Check sheet for the modelled part. Datum: model origin and axes. Units: mm. Face numbers are marked on the shaded views. A direction names the side the tool comes from. Round coordinates to 2 decimals unless told otherwise and drop trailing zeros. Order: outer loops, then holes, each group sorted by start corner. A loop starts at its lowest first (then second) coordinate and runs counter-clockwise, first axis right, second up.
```python
from build123d import *

# Parameters (mm, degrees)
SKETCH2_W               = 1.2
SKETCH2_H               = 2.96832053
CUT_EXTRUDE1_DEPTH      = 3.35
CUT_EXTRUDE1_DEPTH_BACK = 3.35
CHAMFER_1_SIZE          = 0.2


with BuildPart() as part:
    # Sketch1 → Revolve1 (revolve)
    with BuildSketch(Plane(origin=(0, 0, 0), x_dir=(0, 0, -1), z_dir=(1, 0, 0))):
        with BuildLine():
            Line((1.5, -10), (0, -10))
            Line((0, -10), (0, 2))
            Line((0, 2), (1.6, 2))
            ThreePointArc((1.6, 2), (2.130330086, 1.780330086), (2.35, 1.25))
            Line((2.35, 1.25), (2.35, 0))
            Line((2.35, 0), (1.5, 0))
            Line((1.5, 0), (1.5, -10))
        make_face()
    revolve(axis=Axis((0, -26.35, 0), (0, 1, 0)))

    # Sketch2 → Cut-Extrude1 (cut, two sides)
    with BuildSketch(Plane(origin=(0, 0, 0), x_dir=(0, 0, -1), z_dir=(1, 0, 0))) as cut_extrude1_sk:
        with Locations((0.15, 2.515839735)):
            Rectangle(SKETCH2_W, SKETCH2_H)
    extrude(amount=CUT_EXTRUDE1_DEPTH, mode=Mode.SUBTRACT)
    extrude(cut_extrude1_sk.sketch, amount=-CUT_EXTRUDE1_DEPTH_BACK, mode=Mode.SUBTRACT)

    # Фаска1
    chamfer_1_edges = [part.edges().sort_by_distance(p)[0] for p in [
        (0, -10, 1.5),
    ]]
    chamfer(chamfer_1_edges, length=CHAMFER_1_SIZE)


solid = part.part
```
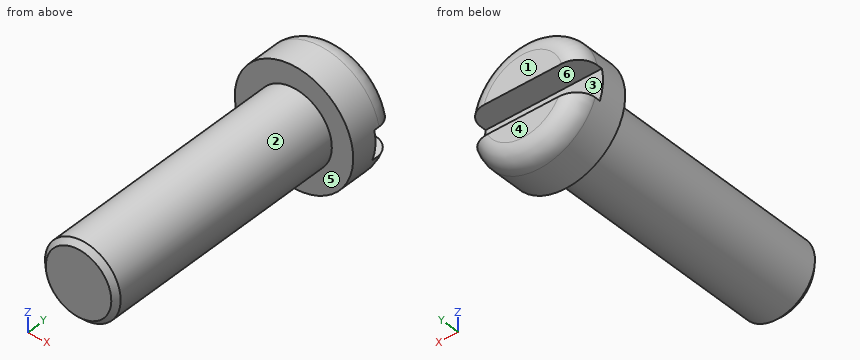
Item 1: Sectioned sample at D-D (y = 0.75). Record the cut outline in (x, z).
Answer:
outline: circle Ø4.7 at (0, 0)
Item 2: Sectioned sample at C-C (y = -7.5). Record the cut outline in (x, z), and give its area (3 significant figures).
Answer:
outline: circle Ø3 at (0, 0)
area: 7.07 mm2
Item 3: Sectioned sample at B-B (x = 0). Record the cut outline in (y, z).
Answer:
outline: (-10, -1.3) - (-9.8, -1.5) - (0, -1.5) - (0, -2.35) - (1.25, -2.35) arc R0.75 ccw to (2, -1.6) - (2, -0.75) - (1.03, -0.75) - (1.03, 0.45) - (2, 0.45) - (2, 1.6) arc R0.75 ccw to (1.25, 2.35) - (0, 2.35) - (0, 1.5) - (-9.8, 1.5) - (-10, 1.3) - close
Item 4: Release check for a two-part mould opening along Z. For the marked faces 1, 2 and 3 record: released by +Z, released by -Z, zero draft, split by the parting line, or undercut.
Answer:
face 1: zero draft
face 2: split by the parting line
face 3: undercut
Item 5: Scan lines: line 1 along Y through (x, z) = (-1.9, -0.3); line 2 along Z through (x, y) = (-0.35, 1.5); line 3 along Z through (x, y) = (-1.5, 0.5). Record each from-to range of solid material in increasing order.
Answer:
line 1: y = 0 to 1.03
line 2: z = -2.28 to -0.75, 0.45 to 2.28
line 3: z = -1.81 to 1.81
Item 6: Access from +Z, -Z, +X, -X, +Y, -Y to the whole of each face (thin tool, end or side, straight path). Record for the marked faces 4, 5 and 6.
Answer:
face 4: +Z, -Z, +X, -X, +Y
face 5: -Y
face 6: +X, -X, +Y
Item 7: Go/stop test with flat-tipped pins: P1, Ø1.5, axis at x = 1, y = -4, coming from the -Z side; P2, Ø1, axis at x = -1, y = -6, coming from the +Z side. Record where each tip stops, or that it passes through.
Answer:
P1: stops at z = -1.48
P2: stops at z = 1.41
Item 8: Sectioned sample at A-A (z = 0). Record the cut outline in (x, y), and give its area (3 significant figures).
Answer:
outline: (-2.35, 0) - (-1.5, 0) - (-1.5, -9.8) - (-1.3, -10) - (1.3, -10) - (1.5, -9.8) - (1.5, 0) - (2.35, 0) - (2.35, 1.03) - (-2.35, 1.03) - close
area: 34.8 mm2
